Work out the finished part from the listing and answer in its coordinate system (mm). Face numbers are marked on the shaded views. A direction names the side the tool comes from. Coordinates: 2 decimals unless noted, no trailing zeros. Order: outer loops, then holes, each group sorted by start corner. A loop starts at its lowest first (then second) coordinate and runs counter-clockwise, first axis right, second up. Notation, with made-up numbers: (-4.5, 18) - (15.5, 18) arc R30 ccw to (15.5, 49) - close; hole circle Ø9 at (-9.75, 70). An arc over 180 degrees is marked (long way). Answer as a JSON object with one key per item and string values. Group by question number.
1) Section A-A (x = 0) is taken. Give the vertices of the cut face in (y, z), plus the area to 3 significant figures.
2) Section D-D (z = 80) is taken. Give the vertices of the cut face in (x, y).
3) Section C-C (y = -7.99) is taken. Give the vertices of the cut face in (x, z), plus the area to 3 significant figures.
4) Section B-B (y = 0) is taken. Give the vertices of the cut face in (x, z), plus the area to 3 significant figures.
5) Each of these flat-tipped pins is pushed along its axis until it touches: P1, Ø1.5, axis at x = -5.5, y = -2, coming from the +Z side; P2, Ø10, axis at y = -4.5, z = 68.5, coming from the +X side; P3, Ø4, axis at x = 0, z = 95, coming from the -Y side. Where does it stop, or does it pass through?
6) Find the intervals of material crossed by line 1 along Z through (x, y) = (0, -9.5); line 2 along Z through (x, y) = (-16, 0.5); line 3 along Z through (x, y) = (13.5, -1), in increasing order.
7) A tool of negligible diameter and unlimited length cuts with its end or side. For the marked faces 1, 2 and 3, from which of +Z, -Z, +X, -X, +Y, -Y can it reach the whole face along a straight path? Write none if from no direction.
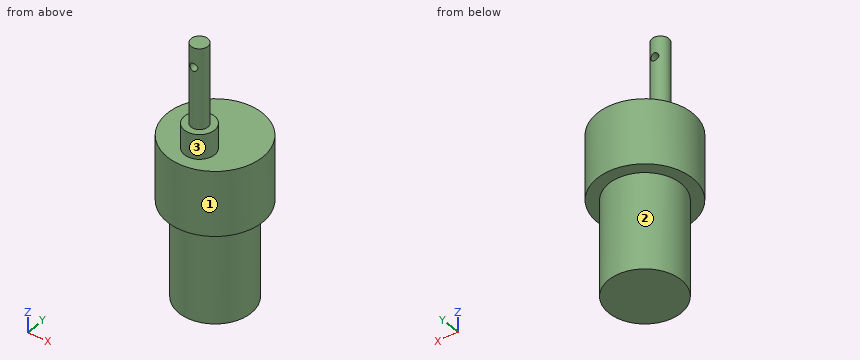
from build123d import *

# Parameters (mm, degrees)
SKETCH6_R           = 13.86
BOSS_EXTRUDE4_DEPTH = 62
SKETCH7_R           = 18.28
BOSS_EXTRUDE5_DEPTH = 25
SKETCH8_R           = 5.79
BOSS_EXTRUDE6_DEPTH = 9.5
SKETCH9_R           = 3.25
BOSS_EXTRUDE7_DEPTH = 31
SKETCH13_R          = 1.5
CUT_EXTRUDE1_DEPTH  = 20


with BuildPart() as part:
    # Sketch6 → Boss-Extrude4 (new body)
    with BuildSketch(Plane.XY):
        Circle(SKETCH6_R)
    extrude(amount=BOSS_EXTRUDE4_DEPTH)

    # Sketch7 → Boss-Extrude5 (add)
    with BuildSketch(Plane.XY.offset(37)):
        Circle(SKETCH7_R)
    extrude(amount=BOSS_EXTRUDE5_DEPTH)

    # Sketch8 → Boss-Extrude6 (add)
    with BuildSketch(Plane.XY.offset(62)):
        with Locations((0, -7.99)):
            Circle(SKETCH8_R)
    extrude(amount=BOSS_EXTRUDE6_DEPTH)

    # Sketch9 → Boss-Extrude7 (add)
    with BuildSketch(Plane.XY.offset(71.5)):
        with Locations((0, -7.99)):
            Circle(SKETCH9_R)
    extrude(amount=BOSS_EXTRUDE7_DEPTH)

    # Sketch13 → Cut-Extrude1 (cut)
    with BuildSketch(Plane(origin=(0, 0, 0), x_dir=(1, 0, 0), z_dir=(0, 1, 0))):
        with Locations((0, -95)):
            Circle(SKETCH13_R)
    extrude(amount=-CUT_EXTRUDE1_DEPTH, mode=Mode.SUBTRACT)


solid = part.part
Report:
{
 "1": {"outline": "(-18.28, 37) - (-13.86, 37) - (-13.86, 0) - (13.86, 0) - (13.86, 37) - (18.28, 37) - (18.28, 62) - (-2.2, 62) - (-2.2, 71.5) - (-4.74, 71.5) - (-4.74, 93.5) - (-11.24, 93.5) - (-11.24, 71.5) - (-13.78, 71.5) - (-13.78, 62) - (-18.28, 62) - close; (-11.24, 96.5) - (-4.74, 96.5) - (-4.74, 102.5) - (-11.24, 102.5) - close", "area": "2,230 mm²"},
 "2": {"outline": "circle Ø6.5 at (0, -7.99)"},
 "3": {"outline": "(-16.44, 37) - (-11.33, 37) - (-11.33, 0) - (11.33, 0) - (11.33, 37) - (16.44, 37) - (16.44, 62) - (5.79, 62) - (5.79, 71.5) - (3.25, 71.5) - (3.25, 102.5) - (-3.25, 102.5) - (-3.25, 71.5) - (-5.79, 71.5) - (-5.79, 62) - (-16.44, 62) - close; hole circle Ø3 at (0, 95)", "area": "1,960 mm²"},
 "4": {"outline": "(-18.28, 37) - (-13.86, 37) - (-13.86, 0) - (13.86, 0) - (13.86, 37) - (18.28, 37) - (18.28, 62) - (-18.28, 62) - close", "area": "1,940 mm²"},
 "5": {"P1": "stops at z = 62", "P2": "stops at x = 5.79", "P3": "stops at y = -11.24"},
 "6": {"line 1": "z = 0 to 93.5, 96.5 to 102.5", "line 2": "z = 37 to 62", "line 3": "z = 0 to 62"},
 "7": {"face 1": "+Z, -Z", "face 2": "-Z", "face 3": "+Z"}
}
